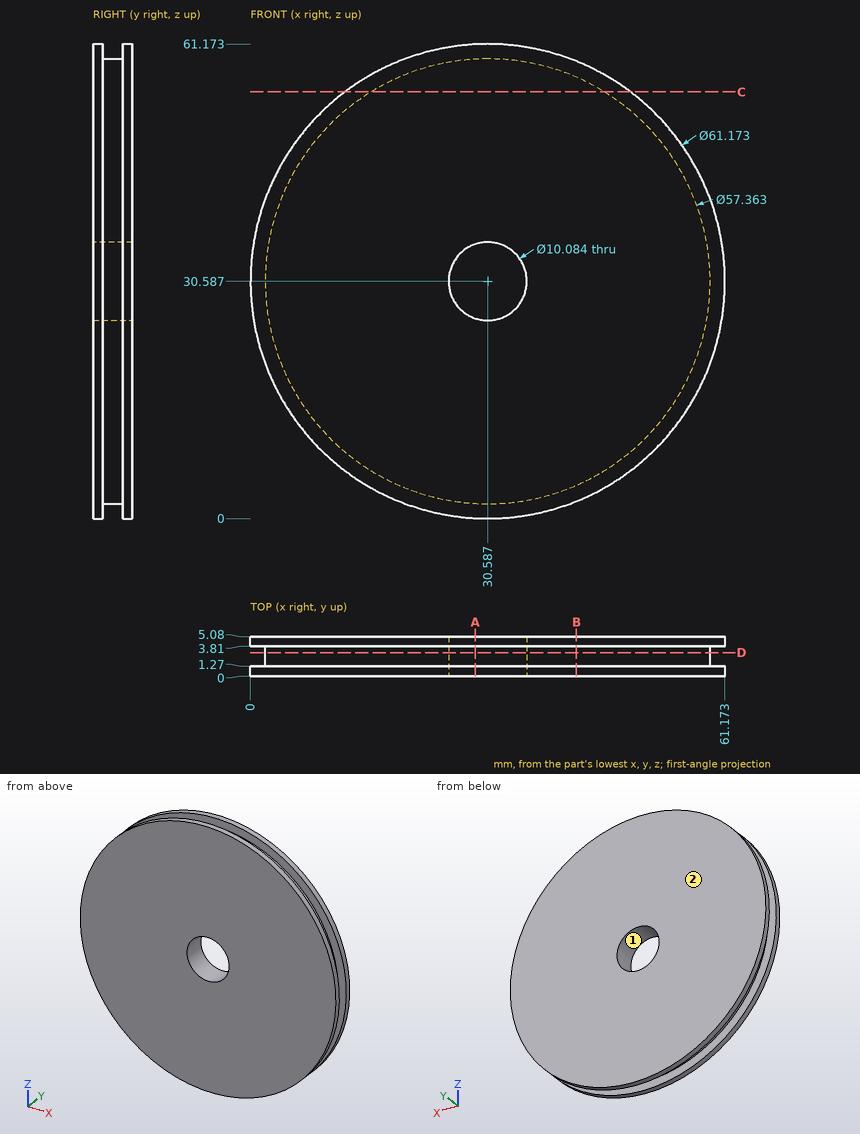
Study the drawing (mm; zero at the part's minimum x, y, z) and answer. Coordinates: 2 decimals unless noted, no trailing zeros. Loops run counter-clockwise (first coordinate to the right, second up) from the corner with the lowest first, then second, coordinate; pieces in that order, holes last. Notation, with made-up numbers: M -34.75,75.25 L 7.25,75.25 A12 ccw 7.25,83.25 Z; hole C 1.25,13 d7. An arc over 180 degrees is marked long. Answer as a JSON object with one key per item and string values. Group by question number.
Item 1: Determine the mould class of the marked faces 1 and 2 for opening direction Z: +Z half, -Z half, draft (parallel to the pull), parting line (faces both ways), or undercut.
Item 2: Section C-C (z = 55) is taken. Write down the section's boundary in (x, y), and give its area (3 significant figures).
Item 3: Section A-A (x = 29) is taken. Write down the section's boundary in (y, z) (1 decimal).
Item 4: Section D-D (y = 3) is taken. Write down the section's boundary in (x, z) (1 decimal), and give its area (3 significant figures).
Item 5: Consider L1, parallel to X at y = 0.7, z = 31.5 (1 decimal); L2, parallel to Z at x = 27.5, y = 1.7 (1 decimal). Determine where each line is inside the solid, lowest interval first.
Item 6: Section B-B (x = 42) is taken. Write down the section's boundary in (y, z).
Item 7: Each of these flat-tipped pins is pushed along its axis until it touches: P1, Ø2, axis at x = 16.5, y = 4.5, coming from the -Z side; P2, Ø1, axis at x = 7, z = 9.5, coming from the +Y side. Where does it stop, or does it pass through?
Solved:
{
 "1": {"face 1": "undercut", "face 2": "draft"},
 "2": {"outline": "M 12.16,0 L 49.01,0 L 49.01,1.27 L 45.64,1.27 L 45.64,3.81 L 49.01,3.81 L 49.01,5.08 L 12.16,5.08 L 12.16,3.81 L 15.53,3.81 L 15.53,1.27 L 12.16,1.27 Z", "area": "170 mm2"},
 "3": {"outline": "M 0,0 L 1.3,0 L 1.3,1.9 L 3.8,1.9 L 3.8,0 L 5.1,0 L 5.1,25.8 L 0,25.8 Z; M 0,35.4 L 5.1,35.4 L 5.1,61.1 L 3.8,61.1 L 3.8,59.2 L 1.3,59.2 L 1.3,61.1 L 0,61.1 Z"},
 "4": {"outline": "C 30.6,30.6 d57.4; hole C 30.6,30.6 d10.1", "area": "2,500 mm2"},
 "5": {"L1": "x = 0 to 25.6, 35.5 to 61.2", "L2": "z = 2.1 to 26.6, 34.6 to 59.1"},
 "6": {"outline": "M 0,2.21 L 1.27,2.21 L 1.27,4.27 L 3.81,4.27 L 3.81,2.21 L 5.08,2.21 L 5.08,58.96 L 3.81,58.96 L 3.81,56.9 L 1.27,56.9 L 1.27,58.96 L 0,58.96 Z"},
 "7": {"P1": "stops at z = 2.94", "P2": "passes through"}
}
